Work out the finished part from the listing and answer in its coordinate system (mm). A direction names the side the tool comes from. Round coordinates to 2 decimals unless told otherwise and drop trailing zeros. Loops run counter-clockwise (first coordinate to the right, second up) from the corner with the lowest first, then second, coordinate; pieces in that order, holes last. Notation, with made-up numbers: M 51.5,59 L 88.5,59 A22 ccw 88.5,96 Z; hole C -7,52.5 d5. An arc over 180 degrees is marked long. One line per item, written item: value.
```python
from build123d import *

# Parameters (mm, degrees)
F1_DEPTH = 25
F2_R     = 5
F3_R     = 3
F4_SIZE  = 5


with BuildPart() as f1:
    # F0 (on Top) → F1 (new body)
    with BuildSketch(Plane.XY):
        Polygon((0, 15), (-3.5, 15), (-3.5, 0), (-9, 0), (-9, -10), (0, -10), (0, 0), (0, 6), (25, 6), (25, 0), (25, -10), (38, -10), (38, 0), (28.7611037493, 0), (28.7611037493, 15), (25, 15), align=None)
    extrude(amount=F1_DEPTH)

    # F2
    f2_edges = [f1.edges().sort_by_distance(p)[0] for p in [
        (-3.5, 15, 12.5),
        (28.761104, 15, 12.5),
        (0, 6, 12.5),
        (25, 6, 12.5),
    ]]
    fillet(f2_edges, radius=F2_R)

    # F3
    f3_edges = [f1.edges().sort_by_distance(p)[0] for p in [
        (28.761104, 0, 12.5),
    ]]
    fillet(f3_edges, radius=F3_R)

    # F4
    f4_edges = [f1.edges().sort_by_distance(p)[0] for p in [
        (38, -10, 12.5),
    ]]
    chamfer(f4_edges, length=F4_SIZE)


solid = f1.part
```
1) Find section A-A (y = -3.5). Give the vertices of the cut face in (x, z), then the cut area to 3 significant figures.
Check values:
outline: M -9,0 L 0,0 L 0,25 L -9,25 Z; M 25,0 L 38,0 L 38,25 L 25,25 Z
area: 550 mm2
2) Find the intervals of material crossed by probe 1 along X at (y, z) = (-1, 10.5); probe 2 along Y at (x, z) = (12, 7.25); probe 3 along Y at (x, z) = (-6, 15), in increasing order. Write a range as from..to.
Check values:
probe 1: -9..0, 25..38
probe 2: 6..15
probe 3: -10..0
3) Find section C-C (y = -6.5). Give the vertices of the cut face in (x, z).
Check values:
outline: M -9,0 L 0,0 L 0,25 L -9,25 Z; M 25,0 L 36.5,0 L 36.5,25 L 25,25 Z
4) The mould has two halves that part along X. Classify faces 1 (the face through (29.62, 0.9, 12.68)), 2 (the face through (0, -5, 12)), 3 (the face through (29, -10, 12)): +X half, -X half, draft (parallel to the pull), parting line (faces both ways), or undercut.
Check values:
face 1: +X half
face 2: undercut
face 3: draft
5) Each of these flat-tipped pins is pushed along its axis until it touches: pin 1 (7 mm diameter, centred on x = 36, z = 17.5, fed in from +Y); pin 2 (6 mm diameter, centred on y = 11, z = 12, fed in from -X); pin 3 (2 mm diameter, centred on y = 7.5, z = 6.5, fed in from +X). Where does it stop, or does it pass through?
Check values:
pin 1: y = 0
pin 2: x = -3.5
pin 3: x = 28.76
6) For faces 4 (the face through (-3.5, 5, 12)), 5 (the face through (28.761, 6, 12)), 6 (the face through (23, 5, 13)), determine the directions among +Z, -Z, +X, -X, +Y, -Y from which every point of the face is accessible in a straight line to the end or side of a thin tool.
Check values:
face 4: +Z, -Z, -X, +Y
face 5: +Z, -Z, +X, +Y
face 6: +Z, -Z, -Y
7) Find section D-D (x = -4). Give the vertices of the cut face in (y, z), then the cut area to 3 significant figures.
Check values:
outline: M -10,0 L 0,0 L 0,25 L -10,25 Z
area: 250 mm2
8) Find section B-B (z = 7.75). Give the vertices of the cut face in (x, y).
Check values:
outline: M -9,-10 L 0,-10 L 0,1 A5 cw 5,6 L 20,6 A5 cw 25,1 L 25,-10 L 33,-10 L 38,-5 L 38,0 L 31.76,0 A3 cw 28.76,3 L 28.76,10 A5 ccw 23.76,15 L 1.5,15 A5 ccw -3.5,10 L -3.5,0 L -9,0 Z
